```python
from build123d import *

# Parameters (mm, degrees)
SKETCH2_W               = 40
SKETCH2_H               = 40
CUT_EXTRUDE1_DEPTH      = 4.2
CUT_EXTRUDE1_DEPTH_BACK = 4.2


with BuildPart() as part:
    # Sketch1 → Revolve1 (revolve)
    with BuildSketch(Plane.XY):
        Polygon((0, 0), (4.95, 0), (10.921281292, -1.6), (4.95, -3.2), (0, -3.2), align=None)
    revolve(axis=Axis((0, -3.2, 0), (0, 1, 0)))

    # Sketch2 → Cut-Extrude1 (cut, two sides)
    with BuildSketch(Plane(origin=(0, 0, 0), x_dir=(1, 0, 0), z_dir=(0, 1, 0))) as cut_extrude1_sk:
        Rectangle(SKETCH2_W, SKETCH2_H)
        Polygon((-5, -2.886751346), (0, -5.773502692), (5, -2.886751346), (5, 2.886751346), (0, 5.773502692), (-5, 2.886751346), align=None, mode=Mode.SUBTRACT)
    extrude(amount=CUT_EXTRUDE1_DEPTH, mode=Mode.SUBTRACT)
    extrude(cut_extrude1_sk.sketch, amount=-CUT_EXTRUDE1_DEPTH_BACK, mode=Mode.SUBTRACT)

    # Sketch3 → Cut-Revolve1 (revolve, cut)
    with BuildSketch(Plane.XY):
        Polygon((0, 0), (3, 0), (2.4585, -0.5415), (2.4585, -2.6585), (3, -3.2), (0, -3.2), align=None)
    revolve(axis=Axis((0, -3.2, 0), (0, 1, 0)), mode=Mode.SUBTRACT)


solid = part.part
```
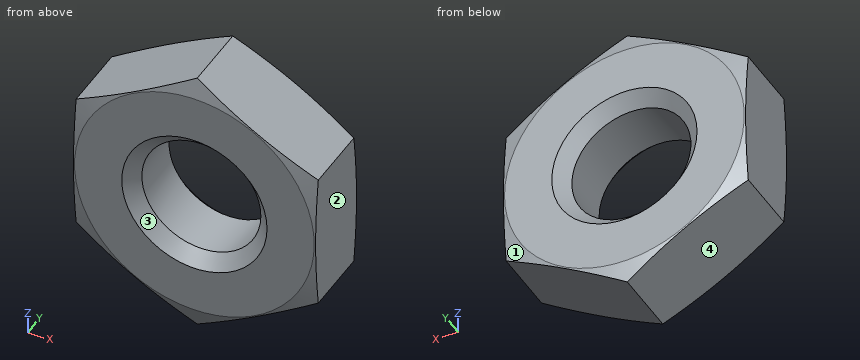
CAD build for the part. Positions are in the model's coordinates, mm. Face numbers are marked on the shaded views. Round coordinates to 2 decimals unless told otherwise and drop trailing zeros. Write each loop counter-clockwise with the first axis right and the second up, starting at its lowest first coordinate (ties: lowest second). Pieces come first, ordered by that corner, then holes. Notation, with made-up numbers: (-31.5, -39) -> (21.5, -39) arc R16 cw to (21.5, -34) -> close; hole circle Ø3 at (38, 67.25). An arc over 180 degrees is marked (long way). Answer in a Markdown table with one row per item. Add a question column.
Item 1: Drop a flat-ended pin along its axis: pin 1 Ø1.5 at (x, z) = (-2, -1.5) entering from -Y. Give the stop position or say it passes through.
Item 2: Mould opens along X. For the marked faces 1, 2, 3 and 4 say: pulls with the +X half, pulls with the -X half, needs draft (parallel to the pull), parting line crosses it, or undercut.
Item 3: Saw through at B-B, the plane y = -0.75. Write the cut outline in (x, z), then the cut area to 3 significant figures.
Item 4: Saw through at A-A, the plane z = 0. Write the cut outline in (x, y), then the cut area to 3 significant figures.
Item 5: Drill centre lines: line 1 (X direction, y = -2, z = 0); line 2 (Z direction, x = 1, y = -0.8); line 3 (X direction, y = -0.3, z = 0.5). Where is each one in solid material? Low to high. Write a range as from..to.
Findings below:
| question | item | result |
|---|---|---|
| 1 | pin 1 | stops at y = -3.2 |
| 2 | face 1 | parting line crosses it |
| 2 | face 2 | pulls with the +X half |
| 2 | face 3 | undercut |
| 2 | face 4 | pulls with the -X half |
| 3 | outline | (-5, -2.89) -> (0, -5.77) -> (5, -2.89) -> (5, 2.89) -> (0, 5.77) -> (-5, 2.89) -> close; hole circle Ø4.92 at (0, 0) |
| 3 | area | 67.6 mm^2 |
| 4 | outline | (-5, -3.19) -> (-4.95, -3.2) -> (-3, -3.2) -> (-2.46, -2.66) -> (-2.46, -0.54) -> (-3, 0) -> (-4.95, 0) -> (-5, -0.01) -> close; (2.46, -2.66) -> (3, -3.2) -> (4.95, -3.2) -> (5, -3.19) -> (5, -0.01) -> (4.95, 0) -> (3, 0) -> (2.46, -0.54) -> close |
| 4 | area | 15.7 mm^2 |
| 5 | line 1 | x = -5..-2.46, 2.46..5 |
| 5 | line 2 | z = -5.2..-2.25, 2.25..5.2 |
| 5 | line 3 | x = -5..-2.65, 2.65..5 |
